Source: CAD feature listing. Evaluate the final solid. Frame: model axes, mm. Give positions to 0.01 mm unless a question says otherwise; leave off trailing zeros. Write each loop counter-clockwise with the first axis right and the second up, starting at its lowest first coordinate (ties: lowest second). Pieces come first, ordered by that corner, then holes. Notation, with made-up numbers: M -17.75,-3 L 21.25,-3 A15 cw 21.25,23 Z; hole C 71.25,59 d8. An arc over 180 degrees is marked long. Answer as a JSON object with one key per item and string values. Group by question number.
```python
from build123d import *

# Parameters (mm, degrees)
F0_W     = 101.6
F0_H     = 76.2
F1_DEPTH = 42.418
F2_R     = 13.442601
F3_DEPTH = 67.564
F4_R     = 10.393123
F5_DEPTH = 93.218
F6_R     = 12.06034
F7_DEPTH = 66.548


with BuildPart() as f1:
    # F0 (on Front) → F1 (new body)
    with BuildSketch(Plane.XZ):
        with Locations((26.758161, 35.611203)):
            Rectangle(F0_W, F0_H)
    extrude(amount=F1_DEPTH)

    # F2 (on Front) → F3 (cut)
    with BuildSketch(Plane.XZ):
        with Locations((19.011559, 53.825341)):
            Circle(F2_R)
    extrude(amount=F3_DEPTH, mode=Mode.SUBTRACT)

    # F4 (on face) → F5 (cut)
    with BuildSketch(Plane.XZ.offset(42.418)):
        with Locations((44.915249, 24.72481)):
            Circle(F4_R)
    extrude(amount=-F5_DEPTH, mode=Mode.SUBTRACT)

    # F6 (on face) → F7 (cut)
    with BuildSketch(Plane.XZ.offset(42.418)):
        with Locations((13.703964, 17.569638)):
            Circle(F6_R)
    extrude(amount=-F7_DEPTH, mode=Mode.SUBTRACT)


solid = f1.part
```
(1) Section A-A, the plane x = 11. Return loops of the section in (y, z).
(2) Contact query for a flat-ended pin moving along its axis: pin 1 Ø21.5 at (x, z) = (13.7, 17.57) entering from +Y. Output: stop coordinate, or through.
(3) Section D-D, the plane x = 41. Return loops of the section in (y, z).
(4) Pull-direction query (X, two-part tool) for faces 1 (the flat face through (26, -42.418, 36)), 2 (the cylindrical face through (17.262, -20.912, 67.154)), 3 (the flat face through (77.558, -21, 35)); classes: pulls with the +X half, pulls with the -X half, needs draft (parallel to the pull), parting line crosses it, or undercut.
(5) Ray query, L1, parallel to Z at x = 18, y = -9; L2, parallel to X at y = -38, z = 23; L3, parallel to Z at x = 15, y = -9.5. Return the intervals inside material, ascending. Write a range as [from, to].
(6) Section B-B, the plane z = 49.5. Return loops of the section in (x, y).
(7) Section C-C, the plane y = -17. Return loops of the section in (x, z), plus the area to 3 significant figures.
Reported:
{
 "1": {"outline": "M -42.42,-2.49 L 0,-2.49 L 0,5.82 L -42.42,5.82 Z; M -42.42,29.32 L 0,29.32 L 0,43.03 L -42.42,43.03 Z; M -42.42,64.62 L 0,64.62 L 0,73.71 L -42.42,73.71 Z"},
 "2": {"pin 1": "passes through"},
 "3": {"outline": "M -42.42,-2.49 L 0,-2.49 L 0,15.1 L -42.42,15.1 Z; M -42.42,34.35 L 0,34.35 L 0,73.71 L -42.42,73.71 Z"},
 "4": {"face 1": "needs draft", "face 2": "undercut", "face 3": "pulls with the +X half"},
 "5": {"L1": "z = [-2.49, 6.3], [28.84, 40.42], [67.23, 73.71]", "L2": "x = [-24.04, 2.94], [24.47, 34.67], [55.16, 77.56]", "L3": "z = [-2.49, 5.58], [29.56, 41], [66.66, 73.71]"},
 "6": {"outline": "M -24.04,-42.42 L 6.28,-42.42 L 6.28,0 L -24.04,0 Z; M 31.74,-42.42 L 77.56,-42.42 L 77.56,0 L 31.74,0 Z"},
 "7": {"outline": "M -24.04,-2.49 L 77.56,-2.49 L 77.56,73.71 L -24.04,73.71 Z; hole C 13.7,17.57 d24.12; hole C 19.01,53.83 d26.89; hole C 44.92,24.72 d20.79", "area": "6,380 mm2"}
}
